from build123d import *

# Parameters (mm, degrees)
SKETCH1_W           = 90
SKETCH1_H           = 20
SKETCH1_R           = 2.5
BOSS_EXTRUDE1_DEPTH = 10
FILLET1_R           = 10


with BuildPart() as part:
    # Sketch1 → Boss-Extrude1 (new body)
    with BuildSketch(Plane.XY):
        Rectangle(SKETCH1_W, SKETCH1_H)
        with Locations((-40, 0.116382556)):
            Circle(SKETCH1_R, mode=Mode.SUBTRACT)
        with Locations((40, 0)):
            Circle(SKETCH1_R, mode=Mode.SUBTRACT)
        Circle(SKETCH1_R, mode=Mode.SUBTRACT)
    extrude(amount=BOSS_EXTRUDE1_DEPTH)

    # Fillet1
    fillet1_edges = [part.edges().sort_by_distance(p)[0] for p in [
        (45, -10, 5),
        (45, 10, 5),
        (-45, -10, 5),
        (-45, 10, 5),
    ]]
    fillet(fillet1_edges, radius=FILLET1_R - 0.0001)  # a hair under: the kernel refuses the full size


solid = part.part
Build history of the part. All positions in model axes, mm. Coordinates: 2 decimals unless noted, no trailing zeros. Write each loop counter-clockwise with the first axis right and the second up, starting at its lowest first coordinate (ties: lowest second). Pieces come first, ordered by that corner, then holes.
(1) Cut at D-D on x = -40. List the corners of the cut face in (y, z), and give its area (3 significant figures).
(2) Cut at C-C on z = 2.25. State how many separate pieces and enclosed holes the cut face has, and give its area (3 significant figures).
(3) Cut at B-B on y = -0.75. List the corners of the cut face in (x, z).
(4) Pin check, flat tip, straight feed: pin 1 Ø4 at (y, z) = (3, 3) entering from -X. Stop position of the tip, or through.
(5) Drill centre lines: line 1 (Y direction, x = -38, z = 6.25); line 2 (Y direction, x = 39.5, z = 3.75); line 3 (X direction, y = -7.5, z = 5.5). Where is each one in solid material? Low to high.
(6) Cut at A-A on x = 0. List the corners of the cut face in (y, z), and give its area (3 significant figures).
(7) Mould opens along X. For faces 1 (the cylindrical face through (-42.15, 6.99, 5.07)), 2 (the flat face through (0, -10, 5)), 3 (the cylindrical face through (-0.54, -2.44, 4.93)) say: pulls with the +X half, pulls with the -X half, needs draft (parallel to the pull), parting line crosses it, or undercut.
Working result:
1. outline: (-8.66, 0) - (-2.38, 0) - (-2.38, 10) - (-8.66, 10) - close; (2.62, 0) - (8.66, 0) - (8.66, 10) - (2.62, 10) - close
1. area: 123 mm2
2. separate pieces: 1
2. enclosed holes: 3
2. area: 1,660 mm2
3. outline: (-44.97, 0) - (-42.35, 0) - (-42.35, 10) - (-44.97, 10) - close; (-37.65, 0) - (-2.38, 0) - (-2.38, 10) - (-37.65, 10) - close; (2.38, 0) - (37.62, 0) - (37.62, 10) - (2.38, 10) - close; (42.38, 0) - (44.97, 0) - (44.97, 10) - (42.38, 10) - close
4. pin 1: stops at x = -44.95
5. line 1: y = -9.54 to -1.38, 1.62 to 9.54
5. line 2: y = -8.93 to -2.45, 2.45 to 8.93
5. line 3: x = -41.61 to 41.61
6. outline: (-10, 0) - (-2.5, 0) - (-2.5, 10) - (-10, 10) - close; (2.5, 0) - (10, 0) - (10, 10) - (2.5, 10) - close
6. area: 150 mm2
7. face 1: pulls with the -X half
7. face 2: needs draft
7. face 3: undercut
